Source: three-view drawing plus pictorial views. Frame: mm from the lowest corner of the part. Round coordinates to 2 decimals unless told otherwise and drop trailing zeros. Loops run counter-clockwise (first coordinate to the right, second up) from the corner with the lowest first, then second, coordinate; pieces in that order, holes last. Notation, with made-up numbers: (5, -12.75) -> (19, -12.75) arc R30 cw to (19, 23.25) -> close; hole circle Ø8 at (4, 18.5). An arc over 180 degrees is marked (long way). Answer as a JSON object with one key per item and string values. Group by question number.
Item 1: Material intervals for line 1 (Z direction, x = 9.5, y = 8); line 2 (Z direction, x = 36, y = 8.75); line 3 (Y direction, x = 28.5, z = 12.25), sorted ascending. Write a range as [from, to].
Item 2: Pin query (flat end, axial travel): pin 1 (1 mm diameter, centred on x = 13.5, z = 3, fed in from -Y); pin 2 (6 mm diameter, centred on x = 28.5, z = 4.5, fed in from -Y); pin 3 (8 mm diameter, centred on x = 29, y = 2, fed in from -Z). Return the tip coordinate at first contact, or that it passes through.
Item 3: Section query A-A on x = 7.5. Return loops of the section in (y, z).
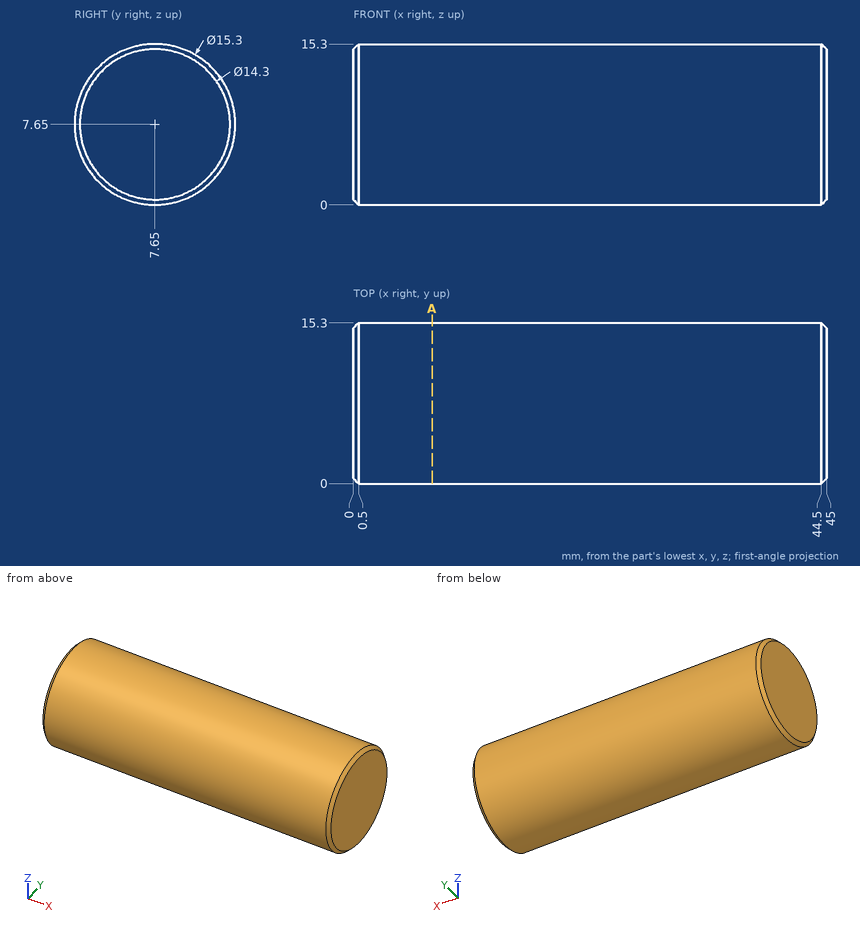
Solved:
{
 "1": {"line 1": "[0.01, 15.29]", "line 2": "[0.08, 15.22]", "line 3": "[1.54, 13.76]"},
 "2": {"pin 1": "y = 1.22", "pin 2": "y = 0", "pin 3": "z = 0.18"},
 "3": {"outline": "circle Ø15.3 at (7.65, 7.65)"}
}
